from build123d import *

# Parameters (mm, degrees)
SM_BASE_FLANGE_1_DEPTH = 270
SKETCH_2_R             = 2
CUT_EXTRUDE_1_DEPTH    = 130
SKETCH_3_R             = 2
CUT_EXTRUDE_2_DEPTH    = 130


# Sheet-metal steps are written as plain solids
with BuildPart() as part:
    # Sketch 1 → Базовая кромка1 (new body)
    with BuildSketch(Plane(origin=(0, 0, 0), x_dir=(1, 0, 0), z_dir=(0, 1, 0))):
        with BuildLine():
            Line((-177.353282485, 51.5), (-219.85622621, 51.5))
            ThreePointArc((-219.85622621, 51.5), (-220.315446329, 51.408655439), (-220.704754348, 51.148528137))
            Line((-220.704754348, 51.148528137), (-250.16981216, 21.683470325))
            ThreePointArc((-250.16981216, 21.683470325), (-250.429939462, 21.294162306), (-250.521284023, 20.834942187))
            Line((-250.521284023, 20.834942187), (-250.521284023, -20.834942187))
            ThreePointArc((-250.521284023, -20.834942187), (-250.429939462, -21.294162306), (-250.16981216, -21.683470325))
            Line((-250.16981216, -21.683470325), (-220.704754348, -51.148528137))
            ThreePointArc((-220.704754348, -51.148528137), (-220.315446329, -51.408655439), (-219.85622621, -51.5))
            Line((-219.85622621, -51.5), (-177.353282485, -51.5))
            Line((-177.353282485, -51.5), (-177.353282485, -52.5))
            Line((-177.353282485, -52.5), (-219.85622621, -52.5))
            ThreePointArc((-219.85622621, -52.5), (-220.698129761, -52.332534972), (-221.411861129, -51.855634919))
            Line((-221.411861129, -51.855634919), (-250.876918941, -22.390577106))
            ThreePointArc((-250.876918941, -22.390577106), (-251.353818994, -21.676845739), (-251.521284023, -20.834942187))
            Line((-251.521284023, -20.834942187), (-251.521284023, 20.834942187))
            ThreePointArc((-251.521284023, 20.834942187), (-251.353818994, 21.676845739), (-250.876918941, 22.390577106))
            Line((-250.876918941, 22.390577106), (-221.411861129, 51.855634919))
            ThreePointArc((-221.411861129, 51.855634919), (-220.698129761, 52.332534972), (-219.85622621, 52.5))
            Line((-219.85622621, 52.5), (-177.353282485, 52.5))
            Line((-177.353282485, 52.5), (-177.353282485, 51.5))
        make_face()
    extrude(amount=SM_BASE_FLANGE_1_DEPTH)

    # Эскиз2 → Вырез-Вытянуть1 (cut)
    with BuildSketch(Plane.XY.offset(52.5)):
        with Locations((-198.604754348, 5)):
            Circle(SKETCH_2_R)
    extrude(amount=-CUT_EXTRUDE_1_DEPTH, mode=Mode.SUBTRACT)

    # Эскиз3 → Вырез-Вытянуть2 (cut)
    with BuildSketch(Plane.ZY.offset(251.521284023)):
        with Locations((0, 5)):
            Circle(SKETCH_3_R)
    extrude(amount=-CUT_EXTRUDE_2_DEPTH, mode=Mode.SUBTRACT)


solid = part.part
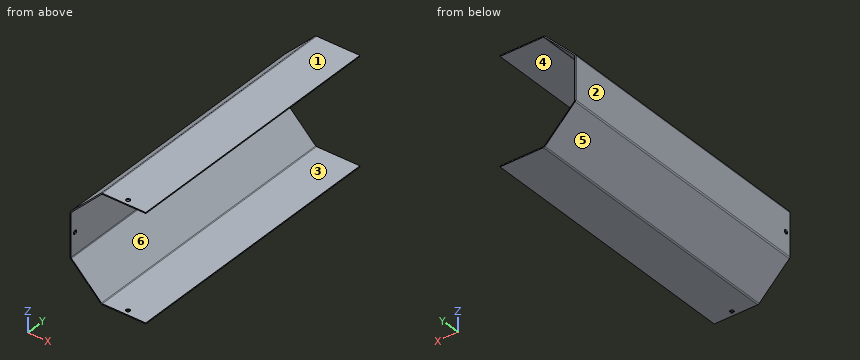
Here's how the part is built. I have some questions about the finished solid (model axes, mm). Face numbers are marked on the shaded views. A direction names the side the tool comes from. Coordinates: 2 decimals unless noted, no trailing zeros. Write each loop counter-clockwise with the first axis right and the second up, starting at its lowest first coordinate (ties: lowest second). Pieces come first, ordered by that corner, then holes.
Item 1: If I drill on line 1 (Z direction, x = -205.5, y = 47); line 2 (X direction, y = 119.5, z = -10); line 3 (Z direction, x = -220.5, y = 177), over which ranges is the centre line in solid material (lowest first)?
Item 2: If we mould it in two halves opening along Z, with no side actions, what happens to the marked faces 1, 2, 3 and 4? For each: +Z half, -Z half, draft (parallel to the pull), parting line (faces both ways), or undercut.
Item 3: I want a section at D-D on x = -236. Write out the boundary of the cut face in (y, z).
Item 4: I want a section at B-B on y = 109. Write out the boundary of the cut face in (x, z).
Item 5: Will these pins go through, and if not, where does the flat tip stop? pin 1 (4.5 mm diameter, centred on x = -198.6, y = 5, fed in from +Z); pin 2 (2.5 mm diameter, centred on y = 5, z = 0, fed in from +X); pin 3 (3 mm diameter, centred on y = 205, z = 6, fed in from +X); pin 4 (1.5 mm diameter, centred on x = -225, y = 182.5, fed in from +Z).
Item 6: On a 3-axis mill with a long thin cutter (end or side, diameter ignored), from which of +Z, -Z, +X, -X, +Y, -Y can I reach the whole of each face in a straight line? I mean the marked faces 5 and 6. Say none if no direction works.
Item 7: I want a section at A-A on x = -184. Write out the boundary of the cut face in (y, z).
Item 8: I want a section at C-C on z = 7.5. Write out the boundary of the cut face in (x, y).
Findings below:
1. line 1: z = -52.5 to -51.5, 51.5 to 52.5
1. line 2: x = -251.52 to -250.52
1. line 3: z = -52.4 to -51.31, 51.31 to 52.4
2. face 1: +Z half
2. face 2: draft
2. face 3: undercut
2. face 4: undercut
3. outline: (0, -37.27) - (270, -37.27) - (270, -35.85) - (0, -35.85) - close; (0, 35.85) - (270, 35.85) - (270, 37.27) - (0, 37.27) - close
4. outline: (-251.52, -20.83) arc R2.2 ccw to (-250.88, -22.39) - (-221.41, -51.86) arc R2.2 ccw to (-219.86, -52.5) - (-177.35, -52.5) - (-177.35, -51.5) - (-219.86, -51.5) arc R1.2 cw to (-220.7, -51.15) - (-250.17, -21.68) arc R1.2 cw to (-250.52, -20.83) - (-250.52, 20.83) arc R1.2 cw to (-250.17, 21.68) - (-220.7, 51.15) arc R1.2 cw to (-219.86, 51.5) - (-177.35, 51.5) - (-177.35, 52.5) - (-219.86, 52.5) arc R2.2 ccw to (-221.41, 51.86) - (-250.88, 22.39) arc R2.2 ccw to (-251.52, 20.83) - close
5. pin 1: stops at z = 52.5
5. pin 2: passes through
5. pin 3: stops at x = -250.52
5. pin 4: stops at z = 49.02
6. face 5: -Z, -X, +Y, -Y
6. face 6: +X, +Y, -Y
7. outline: (0, -52.5) - (270, -52.5) - (270, -51.5) - (0, -51.5) - close; (0, 51.5) - (270, 51.5) - (270, 52.5) - (0, 52.5) - close
8. outline: (-251.52, 0) - (-250.52, 0) - (-250.52, 270) - (-251.52, 270) - close
